Check sheet for the modelled part. Datum: model origin and axes. Units: mm. A direction names the side the tool comes from. Round coordinates to 2 decimals unless told otherwise and drop trailing zeros. Write each loop counter-clockwise with the first axis right and the second up, starting at its lowest first coordinate (ties: lowest second). Pieces come first, ordered by that corner, then holes. Notation, with made-up numbers: (34, -35) -> (51, -35) arc R27 ccw to (51, -8) -> close; hole circle Ø2 at (36.25, 24). An arc over 180 degrees is marked (long way). One line per item, written item: value.
Autodesk Inventor part; units mm, degrees
ref_plane "Work Plane2" through (0, -98, 116) normal (0.5, 0, 0.8660254) x (0, -1, 0)
ref_plane "YZ Plane" through (0, 0, 0) normal (1, 0, 0) x (0, 1, 0)
ref_plane "XZ Plane" through (0, 0, 0) normal (0, 1, 0) x (-1, 0, 0)
sketch "Sketch2" plane through (0, 0, 0) normal (0, 0, 1) x (1, 0, 0)
  line L0 (0, -104) -> (-198, -104)
  line L1 (-198, -104) -> (-198, 104)
  line L2 (-198, 104) -> (0, 104)
  line L3 (0, 104) -> (0, -104)
  point P0 (0, 99)
  point P1 (0, -99)
  point P2 (0, 0)
  dimension "d29" = 198
  dimension "d30" = 208
  dimension "d31" = 5
  dimension "d32" = 5
extrude "Plate2" add sketch "Sketch2" along normal blind 6
sketch "Sketch5" plane through (0, -98, 0) normal (0, -1, 0) x (1, 0, 0)
  line L0 (-198, 0) -> (0, 0)
  line L1 (0, 0) -> (0, 116)
  line L2 (0, 116) -> (-198, 116)
  line L3 (-198, 116) -> (-198, 0)
edge flange "Flange1" height 116 angle 90 thickness 6 bend radius 6 thickness toward (0, -1, 0) relief round relief width 6 relief depth 3 edges at (-99, -104, 6) wall of the first edge with corners at (-198, -98, 0) (0, -98, 0) (0, -98, 116) (-198, -98, 116)
bend "Bend1"
corner "Corner1"
ref_plane "Work Plane2" through (0, -98, 116) normal (0.5, 0, 0.8660254) x (0, -1, 0)
equation "\"d30\" = ChargingHatch_width"
equation "\"d14\" = Thickness"
equation "\"d34\" = BendReliefWidth"
equation "\"d35\" = BendReliefDepth"
equation "\"d36\" = MinimumRemnant"
equation "\"d37\" = TransitionRadius"
equation "\"d38\" = ChargingHatch_hight - Thickness"
equation "\"d40\" = BendRadius"
equation "\"d41\" = CornerReliefSize"
equation "\"d42\" = GapSize"
equation "\"d43\" = JacobiRadiusSize"
equation "\"BendReliefWidth\" = Thickness"
equation "\"BendReliefDepth\" = 0.5 * Thickness"
equation "\"CornerReliefSize\" = 4 * Thickness"
equation "\"MinimumRemnant\" = 2 * Thickness"
equation "\"TransitionRadius\" = BendRadius"
equation "\"JacobiRadiusSize\" = BendRadius"
equation "\"GapSize\" = Thickness"
properties part number "PRS 9672 charging tube 2_D1200 940" material "Steel"
Item 1: Sectioned sample at C-C (y = 25). Enter the section's corners in (x, z), then the cut area to 3 significant figures.
Result set:
outline: (-198, 0) -> (0, 0) -> (0, 6) -> (-198, 6) -> close
area: 1,190 mm^2
Item 2: Sectioned sample at B-B (z = 81). Enter the section's corners in (x, y), then the cut area to 3 significant figures.
Result set:
outline: (-198, -104) -> (0, -104) -> (0, -98) -> (-198, -98) -> close
area: 1,190 mm^2
Item 3: Sectioned sample at A-A (x = -81). Enter the section's corners in (y, z).
Result set:
outline: (-104, 12) arc R12 ccw to (-92, 0) -> (104, 0) -> (104, 6) -> (-92, 6) arc R6 cw to (-98, 12) -> (-98, 116) -> (-104, 116) -> close
Item 4: Material ranges on line 1 along Z through (x, y) = (-167.5, -32); line 2 along Y through (x, z) = (-164, 87), recorded low to high.
Result set:
line 1: 0 to 6
line 2: -104 to -98
Item 5: Depth check by flat-ended pin: pin 1 (1.5 mm diameter, centred on x = -87, y = 41.5, fed in from +Z); pin 2 (5 mm diameter, centred on x = -45, z = 20, fed in from +Y). Enter the tip coordinate at first touch or a pass-through.
Result set:
pin 1: z = 6
pin 2: y = -98
Item 6: Tool access check on faces 1 (the flat face through (-100, 7, 6)), 2 (the flat face through (-198, -47, 2)). Record the directions out of +Z, -Z, +X, -X, +Y, -Y that give a thin tool (end or side, any length) a straight path to the whole face; none if there is none.
Result set:
face 1: +Z, +X, -X, +Y
face 2: +Z, -Z, -X, +Y, -Y
